from build123d import *

# Parameters (mm, degrees)
RESSALTO_EXTRUS_O1_DEPTH = 50
CHANFRO1_SIZE            = 2
ESBO_O2_R                = 3
CORTE_EXTRUS_O1_DEPTH    = 60.039647695
ESBO_O3_R                = 3
CORTE_EXTRUS_O2_DEPTH    = 60.039647695


with BuildPart() as part:
    # Esboço1 → Ressalto-extrusão1 (new body)
    with BuildSketch(Plane.XY):
        Polygon((0, 0), (0, 22.2), (-3.2, 22.2), (-3.2, -3.2), (22.2, -3.2), (22.2, 0), align=None)
    extrude(amount=RESSALTO_EXTRUS_O1_DEPTH)

    # Chanfro1
    chanfro1_edges = [part.edges().sort_by_distance(p)[0] for p in [
        (-1.6, 22.2, 50),
        (22.2, -1.6, 50),
        (22.2, -1.6, 0),
        (-1.6, 22.2, 0),
    ]]
    chamfer(chanfro1_edges, length=CHANFRO1_SIZE)

    # Esboço2 → Corte-extrusão1 (cut, through all)
    with BuildSketch(Plane(origin=(0, 0, 0), x_dir=(1, 0, 0), z_dir=(0, 1, 0))):
        with Locations(Location((11.1, -8, 0), (0, 0, 180))):
            Circle(ESBO_O2_R)
        with Locations(Location((11.1, -42, 0), (0, 0, 180))):
            Circle(ESBO_O2_R)
    extrude(amount=-CORTE_EXTRUS_O1_DEPTH, mode=Mode.SUBTRACT)

    # Esboço3 → Corte-extrusão2 (cut, through all)
    with BuildSketch(Plane(origin=(0, 0, 0), x_dir=(0, 0, -1), z_dir=(1, 0, 0))):
        with Locations(Location((-42, 11.1, 0), (0, 0, 90))):
            Circle(ESBO_O3_R)
        with Locations(Location((-8, 11.1, 0), (0, 0, 90))):
            Circle(ESBO_O3_R)
    extrude(amount=-CORTE_EXTRUS_O2_DEPTH, mode=Mode.SUBTRACT)


solid = part.part
Read the model definition and answer for the solid it produces. Units are mm, in the model's axes. A direction names the side the tool comes from. Give positions to 0.01 mm unless a question says otherwise; leave off trailing zeros. Write each loop counter-clockwise with the first axis right and the second up, starting at its lowest first coordinate (ties: lowest second). Pieces come first, ordered by that corner, then holes. Notation, with made-up numbers: (0.5, 44.5) - (51.5, 44.5) arc R18 ccw to (51.5, 73.5) - close; hole circle Ø3 at (52.5, 65). An arc over 180 degrees is marked (long way). Answer in a Markdown table with one row per item. Add a question column.
Item 1: Find the intervals of material crossed by L1, parallel to Z at x = 11.1, y = -0.9; L2, parallel to X at y = 10.25, z = 11.5, in increasing order.
Item 2: Section C-C, the plane z = 42 is taken. Write down the section's boundary in (x, y).
Item 3: Section A-A, the plane x = 11.1 is taken. Write down the section's boundary in (y, z).
Item 4: Section D-D, the plane x = -0.75 is taken. Write down the section's boundary in (y, z).
Item 5: A tool of negligible diameter and unlimited length cuts with its end or side. For faces 5 (the face through (11, 0, 25)), 6 (the face through (-1.6, 21.2, 49)), from which of +Z, -Z, +X, -X, +Y, -Y can it reach the whole face along a straight path? Write none if from no direction.
Item 6: Determine the mould class of faces 1 (the face through (-3.2, 10, 25)), 2 (the face through (8.24, -1.58, 8.9)), 3 (the face through (21.2, -1.6, 49)), 4 (the face through (-0.2, 4.2, 50)) for opening direction X: pulls with the +X half, pulls with the -X half, needs draft (parallel to the pull), parting line crosses it, or undercut.
Item 7: Flat-ended cylindrical pins translate along their axes: P1, Ø10, axis at x = 9, y = 13, coming from the +Z side; P2, Ø11, axis at x = 9.5, z = 13.5, coming from the +Y side; P3, Ø1, axis at y = 9.5, z = 32, coming from the +X side. Find the tip coordinate at first contact, or state that the pin passes through.
Recorded:
| question | item | result |
|---|---|---|
| 1 | L1 | z = 0 to 5, 11 to 39, 45 to 50 |
| 1 | L2 | x = -3.2 to 0 |
| 2 | outline | (-3.2, -3.2) - (8.1, -3.2) - (8.1, 0) - (0, 0) - (0, 8.1) - (-3.2, 8.1) - close; (-3.2, 14.1) - (0, 14.1) - (0, 22.2) - (-3.2, 22.2) - close; (14.1, -3.2) - (22.2, -3.2) - (22.2, 0) - (14.1, 0) - close |
| 3 | outline | (-3.2, 0) - (0, 0) - (0, 5) - (-3.2, 5) - close; (-3.2, 11) - (0, 11) - (0, 39) - (-3.2, 39) - close; (-3.2, 45) - (0, 45) - (0, 50) - (-3.2, 50) - close |
| 4 | outline | (-3.2, 0) - (20.2, 0) - (22.2, 2) - (22.2, 48) - (20.2, 50) - (-3.2, 50) - close; hole circle Ø6 at (11.1, 8); hole circle Ø6 at (11.1, 42) |
| 5 | face 5 | +Z, -Z, +X, +Y |
| 5 | face 6 | +Z, +X, -X, +Y |
| 6 | face 1 | pulls with the -X half |
| 6 | face 2 | undercut |
| 6 | face 3 | pulls with the +X half |
| 6 | face 4 | needs draft |
| 7 | P1 | passes through |
| 7 | P2 | stops at y = 0 |
| 7 | P3 | stops at x = 0 |
